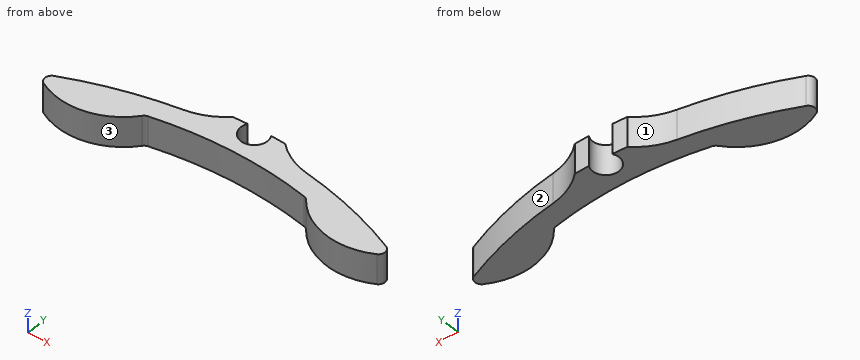
from build123d import *

# Parameters (mm, degrees)
BOSS_EXTRUDE1_DEPTH = 4.5
CUT_EXTRUDE1_DEPTH  = 30.661852099
FILLET1_R           = 10
FILLET2_R           = 1


with BuildPart() as part:
    # Sketch2 → Boss-Extrude1 (new body)
    with BuildSketch(Plane.XY):
        with BuildLine():
            ThreePointArc((-1.74598224, 0.975472203), (0, -2), (1.74598224, 0.975472203))
            ThreePointArc((1.74598224, 0.975472203), (15.131316317, -0.869946427), (27.801563151, -5.564366886))
            ThreePointArc((27.801563151, -5.564366886), (19.812423986, -9.306761236), (11.969278721, -5.267338946))
            ThreePointArc((11.969278721, -5.267338946), (0, -4), (-11.969278721, -5.267338946))
            ThreePointArc((-11.969278721, -5.267338946), (-19.812423986, -9.306761236), (-27.801563151, -5.564366886))
            ThreePointArc((-27.801563151, -5.564366886), (-15.131316317, -0.869946427), (-1.74598224, 0.975472203))
        make_face()
    extrude(amount=BOSS_EXTRUDE1_DEPTH)

    # Sketch3 → Cut-Extrude1 (cut, through all)
    with BuildSketch(Plane.XY.offset(4.5)):
        with BuildLine():
            ThreePointArc((-3.839229312, -1.122638985), (-15.367183828, -2.995958524), (-26.315878496, -7.061563826))
            ThreePointArc((-26.315878496, -7.061563826), (-27.098305385, -6.352245543), (-27.801563151, -5.564366886))
            ThreePointArc((-27.801563151, -5.564366886), (-16.175980809, -1.141817117), (-3.902593708, 0.877361015))
            ThreePointArc((-3.902593708, 0.877361015), (-3.997993987, -0.126665237), (-3.839229312, -1.122638985))
        make_face()
        with BuildLine():
            ThreePointArc((26.315878496, -7.061563826), (15.367183828, -2.995958524), (3.839229312, -1.122638985))
            ThreePointArc((3.839229312, -1.122638985), (3.997993987, -0.126665237), (3.902593708, 0.877361015))
            ThreePointArc((3.902593708, 0.877361015), (16.175980809, -1.141817117), (27.801563151, -5.564366886))
            ThreePointArc((27.801563151, -5.564366886), (27.098305385, -6.352245543), (26.315878496, -7.061563826))
        make_face()
    extrude(amount=-CUT_EXTRUDE1_DEPTH, mode=Mode.SUBTRACT)

    # Fillet1
    # the kernel refuses this fillet: 10 mm, written as the material it adds along each edge
    with BuildSketch(Plane(origin=(-3.839229312, -1.122638985, 4.5), x_dir=(-0.9940877478699028, -0.10857969209269472, 0), z_dir=(0, 0, -1))) as fillet1_piece_1:
        with BuildLine():
            CenterArc((5.852686638, 9.989908799), FILLET1_R, 233.080982265, 34.344798216)
            Line((-0.154169614, 1.995055582), (-0.27430674, 1.835158518))
            ThreePointArc((-0.27430674, 1.835158518), (-0.14972201, 0.99191469), (-0.196921331, 0.034956966))
            Line((-0.196921331, 0.034956966), (0.008982698, -0.199798176))
            ThreePointArc((0.008982698, -0.199798176), (2.701775857, -0.139296277), (5.394569015, -0.199798176))
            Line((5.394569015, -0.199798176), (5.403551713, 0))
        make_face()
    extrude(amount=4.5)
    with BuildSketch(Plane(origin=(3.839229312, -1.122638985, 4.5), x_dir=(0.9940877478699031, -0.10857969209269294, 0), z_dir=(0, 0, -1))) as fillet1_piece_2:
        with BuildLine():
            CenterArc((5.852686638, -9.989908799), FILLET1_R, 92.574219519, 34.344798216)
            Line((-0.154169614, -1.995055582), (-0.27430674, -1.835158518))
            ThreePointArc((-0.27430674, -1.835158518), (-0.14972201, -0.99191469), (-0.196921331, -0.034956966))
            Line((-0.196921331, -0.034956966), (0.008982698, 0.199798176))
            ThreePointArc((0.008982698, 0.199798176), (2.701775857, 0.139296277), (5.394569015, 0.199798176))
            Line((5.394569015, 0.199798176), (5.403551713, 0))
        make_face()
    extrude(amount=4.5)

    # Fillet2
    fillet2_edges = [part.edges().sort_by_distance(p)[0] for p in [
        (11.969278721, -5.267338946, 2.25),
        (-11.969278721, -5.267338946, 2.25),
        (26.315878496, -7.061563826, 2.25),
        (-26.315878496, -7.061563826, 2.25),
    ]]
    fillet(fillet2_edges, radius=FILLET2_R)


solid = part.part
Read the model definition and answer for the solid it produces. Units are mm, in the model's axes. Face numbers are marked on the shaded views. Coordinates: 2 decimals unless noted, no trailing zeros. Loops run counter-clockwise (first coordinate to the right, second up) from the corner with the lowest first, then second, coordinate; pieces in that order, holes last.
Q1. This flat-tipped pin is pushed along its axis until it touches: pin 1 Ø2 at (x, z) = (0.5, 2.5) entering from -Y. Where does it stop, or does it pass through?
Q2. The part is cut by section C-C on y = 0.25. Write down the section's boundary in (x, z), and give its area (3 significant figures).
Q3. The part is cut by section B-B on x = 0. Write down the section's boundary in (y, z), and give its area (3 significant figures).
Q4. The mould has two halves that part along X. Classify the marked faces 1, 2 and 3: +X half, -X half, draft (parallel to the pull), parting line (faces both ways), or undercut.
Q5. Consider probe 1 along Y at (x, z) = (0, 2.45); probe 2 along X at (y, z) = (0, 1.65); probe 3 along X at (y, z) = (-6.5, 0.2). Determine where each line is inside the solid, lowest interval first.
Q6. The part is cut by section A-A on y = -4.5. Write down the section's boundary in (x, z).
Q7. The part is cut by section D-D on y = -2.5. Write down the section's boundary in (x, z), and give its area (3 significant figures).
Results below:
1. pin 1: stops at y = -4.02
2. outline: (-4.64, 0) - (-1.98, 0) - (-1.98, 4.5) - (-4.64, 4.5) - close; (1.98, 0) - (4.64, 0) - (4.64, 4.5) - (1.98, 4.5) - close
2. area: 23.9 mm2
3. outline: (-4, 0) - (-2, 0) - (-2, 4.5) - (-4, 4.5) - close
3. area: 9.00 mm2
4. face 1: -X half
4. face 2: +X half
4. face 3: undercut
5. probe 1: y = -4 to -2
5. probe 2: x = -4.98 to -2, 2 to 4.98
5. probe 3: x = -24.99 to -13.05, 13.05 to 24.99
6. outline: (-20.22, 0) - (-7.54, 0) - (-7.54, 4.5) - (-20.22, 4.5) - close; (7.54, 0) - (20.22, 0) - (20.22, 4.5) - (7.54, 4.5) - close
7. outline: (-13.35, 0) - (13.35, 0) - (13.35, 4.5) - (-13.35, 4.5) - close
7. area: 120 mm2
